```python
from build123d import *

# Parameters (mm, degrees)
EXTRUDE_2_DEPTH          = 13
CUT_EXTRUDE_2_DEPTH      = 86.300937861
CUT_EXTRUDE_2_DEPTH_BACK = 86.300937861
SKETCH_2_R               = 6
SKETCH_2_R_2             = 15
SKETCH_3_W               = 100
SKETCH_3_H               = 100
CUT_EXTRUDE_3_DEPTH      = 3
SKETCH_4_W               = 70
SKETCH_4_H               = 77
CUT_EXTRUDE_4_DEPTH      = 3
FILLET_1_R               = 3


with BuildPart() as part:
    # 스케치1 → 보스-돌출2 (new body)
    with BuildSketch(Plane(origin=(0, 0, 0), x_dir=(1, 0, 0), z_dir=(0, 1, 0))):
        with BuildLine():
            Line((-62, 38.5), (62, 38.5))
            ThreePointArc((62, 38.5), (71.192388155, 34.692388155), (75, 25.5))
            Line((75, 25.5), (75, -25.5))
            ThreePointArc((75, -25.5), (71.192388155, -34.692388155), (62, -38.5))
            Line((62, -38.5), (-62, -38.5))
            ThreePointArc((-62, -38.5), (-71.192388155, -34.692388155), (-75, -25.5))
            Line((-75, -25.5), (-75, 25.5))
            ThreePointArc((-75, 25.5), (-71.192388155, 34.692388155), (-62, 38.5))
        make_face()
    extrude(amount=EXTRUDE_2_DEPTH)

    # 스케치2 → 컷-돌출2 (cut, two sides: drawn at the far end of the back side and taken through both)
    with BuildSketch(Plane(origin=(0, 0, 0), x_dir=(1, 0, 0), z_dir=(0, 1, 0)).offset(-CUT_EXTRUDE_2_DEPTH_BACK)):
        with Locations(Location((-62, 25.5, 0), (0, 0, 270))):
            Circle(SKETCH_2_R)
        with Locations(Location((-62, -25.5, 0), (0, 0, 270))):
            Circle(SKETCH_2_R)
        with Locations(Location((62, -25.5, 0), (0, 0, 270))):
            Circle(SKETCH_2_R)
        with Locations(Location((62, 25.5, 0), (0, 0, 270))):
            Circle(SKETCH_2_R)
        with Locations(Location((0, 0, 0), (0, 0, 270))):
            Circle(SKETCH_2_R_2)
    extrude(amount=CUT_EXTRUDE_2_DEPTH + CUT_EXTRUDE_2_DEPTH_BACK, mode=Mode.SUBTRACT)

    # 스케치3 → 컷-돌출3 (cut)
    with BuildSketch(Plane(origin=(0, 13, 0), x_dir=(1, 0, 0), z_dir=(0, 1, 0))):
        with Locations((85, 0)):
            Rectangle(SKETCH_3_W, SKETCH_3_H)
        with Locations((-85, 0)):
            Rectangle(SKETCH_3_W, SKETCH_3_H)
    extrude(amount=-CUT_EXTRUDE_3_DEPTH, mode=Mode.SUBTRACT)

    # 스케치4 → 컷-돌출4 (cut)
    with BuildSketch(Plane.XZ):
        Rectangle(SKETCH_4_W, SKETCH_4_H)
    extrude(amount=-CUT_EXTRUDE_4_DEPTH, mode=Mode.SUBTRACT)

    # 필렛1
    fillet_1_edges = [part.edges().sort_by_distance(p)[0] for p in [
        (-35, 3, 0),
        (35, 3, 0),
    ]]
    fillet(fillet_1_edges, radius=FILLET_1_R - 0.0001)  # a hair under: the kernel refuses the full size


solid = part.part
```
CAD build for the part. Positions are in the model's coordinates, mm. A direction names the side the tool comes from. Coordinates: 2 decimals unless noted, no trailing zeros. Order: outer loops, then holes, each group sorted by start corner. A loop starts at its lowest first (then second) coordinate and runs counter-clockwise, first axis right, second up. Notation, with made-up numbers: (75.25, 47) - (115.25, 47) arc R18 cw to (115.25, 75) - close; hole circle Ø5 at (-18, -30). An arc over 180 degrees is marked (long way). Use a Markdown table: item, result. Add a question column.
(1) Which spindle directions (+Z, -Z, +X, -X, +Y, -Y) get a long thin tool onto all of the face, cutting with end or side? Do faces 1 (the face through (-34.14, 2.1, 0.54)), 2 (the face through (35, 12, 1)), 3 (the face through (-35, 12, 1)). Say none if no direction does.
(2) Saw through at D-D (x = -64). Give the cut face in (y, z).
(3) Pull direction Z, two halves, no side cores. Call faces 4 (the face through (34.1, 2.14, 0.54)), 5 (the face through (-71.091, 4.93, 34.793)), 6 (the face through (0.66, 7.93, -14.985)), 7 (the face through (71.091, 4.93, -34.793)): +Z half, -Z half, draft (parallel to the pull), parting line (faces both ways), or undercut.
(4) Drill centre lines: line 1 along Z through (x, y) = (-62, 4.25); line 2 along X through (y, z) = (4.25, -25.5); line 3 along X through (y, z) = (8.75, 0). Where is each one in solid material? Low to high. Write a range as [from, to].
(5) Flat gauge pins, fed straight in: pin 1 (15.5 mm diameter, centred on x = 62, z = -25.5, fed in from +Y); pin 2 (3.5 mm diameter, centred on y = 11, z = 5, fed in from +X); pin 3 (11 mm diameter, centred on x = 62, z = 25.5, fed in from +Y); pin 4 (0.9 mm diameter, centred on y = 11, z = 12.5, fed in from -X). Where does each tip first touch, or does it go through?
(6) Saw through at C-C (y = 6.75). Give the cut face in (x, z), then the cut area to 3 significant figures.
(7) Saw through at A-A (x = 0). Give the cut face in (y, z), then the cut area to 3 significant figures.
Solved:
| question | item | result |
|---|---|---|
| 1 | face 1 | +Z, -Z, -Y |
| 1 | face 2 | +Z, -Z, +X, +Y |
| 1 | face 3 | +Z, -Z, -X, +Y |
| 2 | outline | (0, -38.35) - (10, -38.35) - (10, -31.16) - (0, -31.16) - close; (0, -19.84) - (10, -19.84) - (10, 19.84) - (0, 19.84) - close; (0, 31.16) - (10, 31.16) - (10, 38.35) - (0, 38.35) - close |
| 3 | face 4 | draft |
| 3 | face 5 | +Z half |
| 3 | face 6 | undercut |
| 3 | face 7 | -Z half |
| 4 | line 1 | z = [-38.5, -31.5], [-19.5, 19.5], [31.5, 38.5] |
| 4 | line 2 | x = [-75, -68], [-56, 56], [68, 75] |
| 4 | line 3 | x = [-75, -15], [15, 75] |
| 5 | pin 1 | stops at y = 10 |
| 5 | pin 2 | stops at x = 75 |
| 5 | pin 3 | passes through |
| 5 | pin 4 | stops at x = -35 |
| 6 | outline | (-75, -25.5) arc R13 ccw to (-62, -38.5) - (62, -38.5) arc R13 ccw to (75, -25.5) - (75, 25.5) arc R13 ccw to (62, 38.5) - (-62, 38.5) arc R13 ccw to (-75, 25.5) - close; hole circle Ø12 at (-62, -25.5); hole circle Ø12 at (-62, 25.5); hole circle Ø30 at (0, 0); hole circle Ø12 at (62, -25.5); hole circle Ø12 at (62, 25.5) |
| 6 | area | 10,200 mm² |
| 7 | outline | (3, -38.5) - (13, -38.5) - (13, -15) - (3, -15) - close; (3, 15) - (13, 15) - (13, 38.5) - (3, 38.5) - close |
| 7 | area | 470 mm² |
